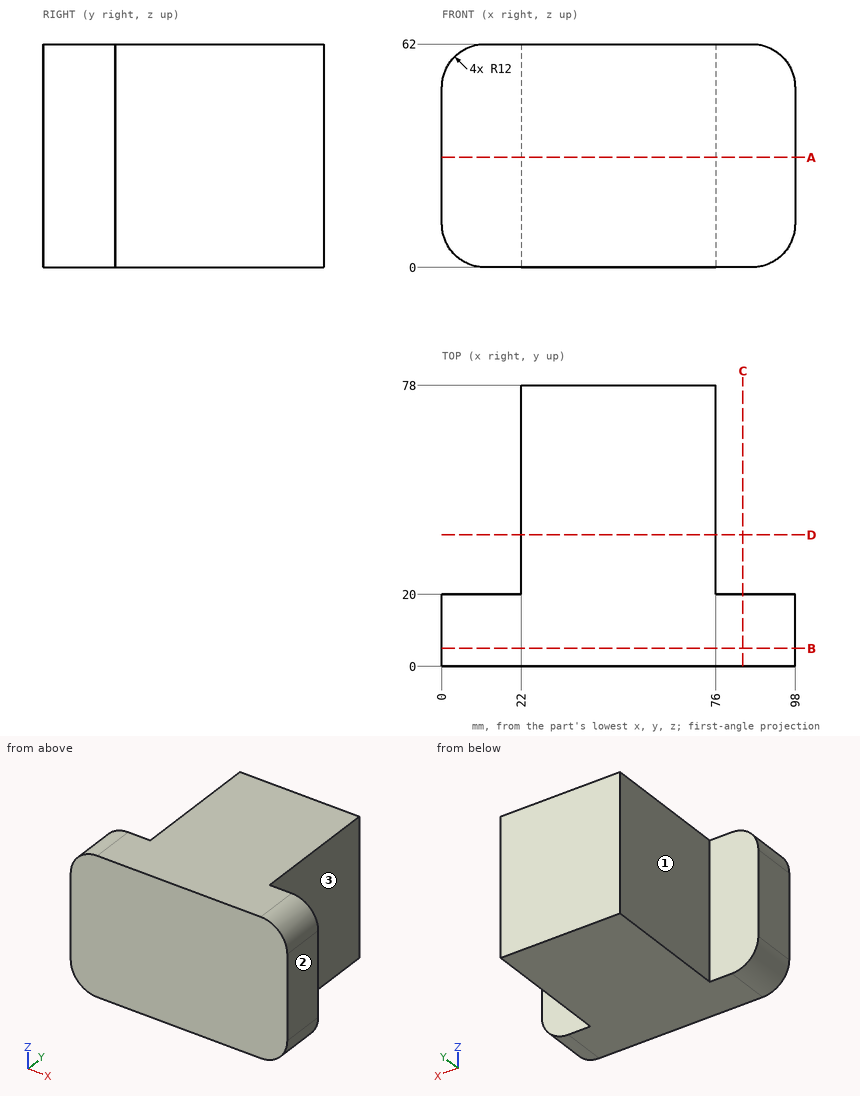
For this review, use the dimensioned drawing (mm, ordinates from the lowest corner) and the shaded views. A direction names the side the tool comes from. Round coordinates to 2 decimals unless told otherwise and drop trailing zeros. Write each loop counter-clockwise with the first axis right and the second up, starting at its lowest first coordinate (ties: lowest second). Pieces come first, ordered by that corner, then holes. Notation, with made-up numbers: (22, 68.5) -> (56, 68.5) arc R33 ccw to (56, 101.5) -> close; hole circle Ø1 at (64, -14). An arc over 180 degrees is marked (long way). Use CSV: the item, a comma, the result in double quotes.
(1) Clearance check with flat-ended pins moving along their axes: P1, Ø11, axis at x = 8, z = 17, coming from the +Y side; P2, Ø6, axis at y = 39, z = 47.5, coming from the -X side; P3, Ø2, axis at x = 19.5, y = 65, coming from the -Z side. State where each tip first meets the part, or that it passes through.
Computed values:
P1,"y = 20"
P2,"x = 22"
P3,"through"
(2) Consider section B-B, the plane y = 5. Give the boundary of the cut face in (x, z).
Computed values:
outline,"(0, 12) arc R12 ccw to (12, 0) -> (86, 0) arc R12 ccw to (98, 12) -> (98, 50) arc R12 ccw to (86, 62) -> (12, 62) arc R12 ccw to (0, 50) -> close"
(3) Consider section C-C, the plane x = 83.5. Give the boundary of the cut face in (y, z).
Computed values:
outline,"(0, 0) -> (20, 0) -> (20, 62) -> (0, 62) -> close"
(4) For the marked faces 1, 2 and 3, list the 3-axis set-ups (+Z, -Z, +X, -X, +Y, -Y) from which the entire face can be reached by the end or side of a thin tool; tool diameter is ignored.
Computed values:
face 1,"+Z, -Z, -X, +Y"
face 2,"+Z, -Z, +X, +Y, -Y"
face 3,"+Z, -Z, +X, +Y"
(5) To check wall thickness, follow L1, parallel to Y at x = 15, z = 58.5; L2, parallel to X at y = 61, z = 33.5. State the ranges of each line that lie inside material, in increasing order. Write a range as [from, to].
Computed values:
L1,"[0, 20]"
L2,"[22, 76]"
(6) Consider section A-A, the plane z = 30.5. Give the boundary of the cut face in (x, y), plus the area to 3 significant figures.
Computed values:
outline,"(0, 0) -> (98, 0) -> (98, 20) -> (76, 20) -> (76, 78) -> (22, 78) -> (22, 20) -> (0, 20) -> close"
area,"5,090 mm²"
(7) Consider section D-D, the plane y = 36.5. Give the boundary of the cut face in (x, z), plus the area to 3 significant figures.
Computed values:
outline,"(22, 0) -> (76, 0) -> (76, 62) -> (22, 62) -> close"
area,"3,350 mm²"
